The listing builds one solid part. Answer for the finished solid, in the listing's coordinates (mm). Face numbers are marked on the shaded views. A direction names the side the tool comes from. Give positions to 0.01 mm unless a question says otherwise; leave off trailing zeros. Write each loop counter-clockwise with the first axis right and the second up, starting at its lowest first coordinate (ties: lowest second). Pieces come first, ordered by that corner, then holes. Notation, with made-up numbers: (72.5, 17.25) - (118.5, 17.25) arc R20 cw to (118.5, 38.25) - close; hole circle Ø3 at (-38, 5.25). An arc over 180 degrees is marked (long way). Answer as CSV lines item,"result". Start each with the question number.
(1) Find section A-A (x = 9.2). Write down the section's boundary in (y, z) (3 decimals).
(2) Find section D-D (x = 14.5). Write down the section's boundary in (y, z) (3 decimals), then the cut area to 3 significant figures.
(3) Find section C-C (z = 0). Write down the section's boundary in (x, y), then the cut area to 3 significant figures.
(4) For the marked faces 4, 5 and 6, determine the directions among +Z, -Z, +X, -X, +Y, -Y from which every point of the face is accessible in a straight line to the end or side of a thin tool.
(5) Each of these flat-tipped pins is pushed along its axis until it touches: pin 1 Ø1.5 at (x, z) = (-10, -0.5) entering from +Y; pin 2 Ø1.5 at (x, y) = (-2.5, 1) entering from -Z. Where does it stop, or does it pass through?
(6) Straight lines are drawn through the part: probe 1 along Y at (x, z) = (9.2, 1); probe 2 along X at (y, z) = (0, -1); probe 3 along Y at (x, z) = (-2.5, -1). For each, find the intervals that lie inside material, in ascending order.
(7) Find section B-B (y = 0). Write down the section's boundary in (x, z) (3 decimals).
(8) For a pull along Y with two mould halves and no side action, classify the marked faces 1, 2 and 3 as pulls with the +Y half, pulls with the -Y half, needs draft (parallel to the pull), parting line crosses it, or undercut.
from build123d import *

# Parameters (mm, degrees)
F1_DEPTH      = 3.375
F1_DEPTH_BACK = 3.375
F2_R          = 2.4
F3_DEPTH      = 18.5
F4_T1_DEPTH   = 21.2682356522


# Not quite as in the source:
# - a fillet or chamfer that OpenCascade refuses, or shapes differently, is made with other operations: its cross-section is extruded or revolved along the edge and cut away or added


with BuildPart() as f1:
    # F0 (on Top) → F1 (new body, two sides)
    with BuildSketch(Plane.XY) as f1_sk:
        with BuildLine():
            Line((16.5, 3.5), (0, 3.5))
            Line((0, 3.5), (0, 2.35))
            Line((0, 2.35), (0, -2.35))
            Line((0, -2.35), (0, -3.5))
            Line((0, -3.5), (16.5, -3.5))
            Line((16.5, -3.5), (16.5, -1.85))
            Line((16.5, -1.85), (13.2, -1.15))
            Line((13.2, -1.15), (9.8304760106, -1.25))
            ThreePointArc((9.8304760106, -1.25), (7.8, 0), (9.8304760106, 1.25))
            Line((9.8304760106, 1.25), (13.2, 1.15))
            Line((13.2, 1.15), (16.5, 1.85))
            Line((16.5, 1.85), (16.5, 3.5))
        make_face()
    extrude(amount=F1_DEPTH)
    extrude(f1_sk.sketch, amount=-F1_DEPTH_BACK)

    # F2 (on face) → F3 (join)
    with BuildSketch(Plane(origin=(0, 0, 0), x_dir=(0, -1, 0), z_dir=(-1, 0, 0))):
        Circle(F2_R)
    extrude(amount=F3_DEPTH)

    # F4: fillet of radius 3.3798989873 on 2 edges, made by hand

    # F4_s2 → F4_t1 (cut)
    with BuildSketch(Plane.XY.offset(-10.6341178261)):
        with BuildLine():
            ThreePointArc((13.5963528696, -3.5), (15.2662081521, -3.0586891941), (16.5, -1.85))
            Line((16.5, -1.85), (16.5, -3.5))
            Line((16.5, -3.5), (13.5963528696, -3.5))
        make_face()
        with BuildLine():
            ThreePointArc((16.5, 1.85), (15.2662081521, 3.0586891941), (13.5963528696, 3.5))
            Line((13.5963528696, 3.5), (16.5, 3.5))
            Line((16.5, 3.5), (16.5, 1.85))
        make_face()
    extrude(amount=F4_T1_DEPTH, mode=Mode.SUBTRACT)


solid = f1.part
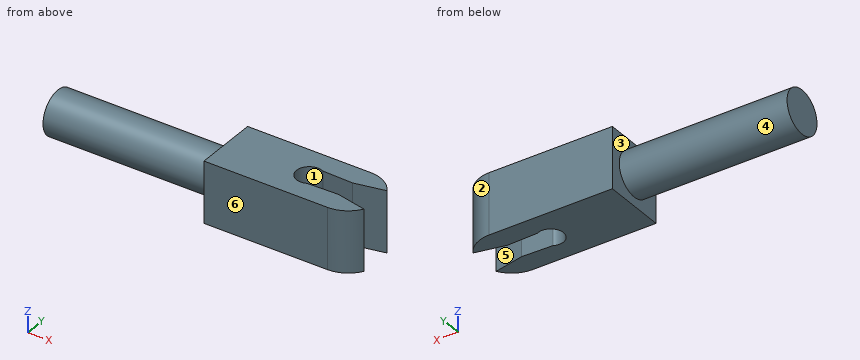
Result set:
1,outline,"(-3.5, -3.375) - (-1.4, -3.375) - (-1.4, 3.375) - (-3.5, 3.375) - close; (1.4, -3.375) - (3.5, -3.375) - (3.5, 3.375) - (1.4, 3.375) - close"
2,outline,"(-3.377, -3.375) - (-1.426, -3.375) - (-1.426, 3.375) - (-3.377, 3.375) - close; (1.426, -3.375) - (3.377, -3.375) - (3.377, 3.375) - (1.426, 3.375) - close"
2,area,"26.3 mm^2"
3,outline,"(-18.5, -2.4) - (0, -2.4) - (0, -3.5) - (13.6, -3.5) arc R3.38 ccw to (16.5, -1.85) - (13.2, -1.15) - (9.83, -1.25) arc R1.4 cw (long way) to (9.83, 1.25) - (13.2, 1.15) - (16.5, 1.85) arc R3.38 ccw to (13.6, 3.5) - (0, 3.5) - (0, 2.4) - (-18.5, 2.4) - close"
3,area,"179 mm^2"
4,face 4,"-X"
4,face 5,"+Z, -Z, +X"
4,face 6,"+Z, -Z, +X, -X, -Y"
5,pin 1,"y = 2.4"
5,pin 2,"z = -2.39"
6,probe 1,"-3.5 to -1.4, 1.4 to 3.5"
6,probe 2,"-18.5 to 7.8"
6,probe 3,"-2.18 to 2.18"
7,outline,"(-18.5, -2.4) - (0, -2.4) - (0, -3.375) - (7.8, -3.375) - (7.8, 3.375) - (0, 3.375) - (0, 2.4) - (-18.5, 2.4) - close"
8,face 1,"undercut"
8,face 2,"pulls with the +Y half"
8,face 3,"needs draft"
